For this review, take the finished solid that the model builds, in its own axes (mm). A direction names the side the tool comes from. Coordinates: 2 decimals unless noted, no trailing zeros. Loops run counter-clockwise (first coordinate to the right, second up) from the corner with the lowest first, then second, coordinate; pieces in that order, holes last. Notation, with made-up numbers: M -32.75,52.5 L 3.25,52.5 A3 ccw 3.25,56.5 Z; hole C -12,2.25 d2. An arc over 180 degrees is marked long. Write item = value, one per line.
from build123d import *

# Parameters (mm, degrees)
SKETCH_1_W          = 5.6
SKETCH_1_H          = 10
EXTRUDE_1_DEPTH     = 8
SKETCH_2_W          = 3.1
SKETCH_2_H          = 5.5
CUT_EXTRUDE_1_DEPTH = 11.970870522
CUT_EXTRUDE_2_REACH = 15.109
SKETCH_3_R          = 1.5
SKETCH_4_R          = 1.5
CUT_EXTRUDE_3_DEPTH = 11.970870522
FILLET_1_R          = 3


with BuildPart() as part:
    # 草图1 → 凸台-拉伸1 (new body)
    with BuildSketch(Plane(origin=(0, 0, 0), x_dir=(1, 0, 0), z_dir=(0, 1, 0))):
        Rectangle(SKETCH_1_W, SKETCH_1_H)
    extrude(amount=EXTRUDE_1_DEPTH)

    # 草图2 → 切除-拉伸1 (cut, through all)
    with BuildSketch(Plane(origin=(2.8, 0, 0), x_dir=(0, 0, -1), z_dir=(1, 0, 0))):
        with Locations((-1, 4)):
            Rectangle(SKETCH_2_W, SKETCH_2_H)
    extrude(amount=-CUT_EXTRUDE_1_DEPTH, mode=Mode.SUBTRACT)

    # 草图3 → 切除-拉伸2 (cut, up to next)
    with BuildSketch(Plane.XY.offset(5), mode=Mode.PRIVATE) as cut_extrude_2_sk1:
        with Locations((0, 4)):
            Circle(SKETCH_3_R)
    cut_extrude_2_tool1 = extrude(cut_extrude_2_sk1.sketch, amount=-CUT_EXTRUDE_2_REACH, mode=Mode.PRIVATE) & part.part
    # 草图3 → 切除-拉伸2 (cut, up to next)
    with BuildSketch(Plane.XY.offset(5), mode=Mode.PRIVATE) as cut_extrude_2_sk2:
        with BuildLine():
            Line((2.8, 5.5), (0, 5.5))
            ThreePointArc((0, 5.5), (1.060660172, 5.060660172), (1.5, 4))
            ThreePointArc((1.5, 4), (1.060660172, 2.939339828), (0, 2.5))
            Line((0, 2.5), (2.8, 2.5))
            Line((2.8, 2.5), (2.8, 5.5))
        make_face()
    cut_extrude_2_tool2 = extrude(cut_extrude_2_sk2.sketch, amount=-CUT_EXTRUDE_2_REACH, mode=Mode.PRIVATE) & part.part
    add(cut_extrude_2_tool1.solids().sort_by_distance((0, 4, 5))[0], mode=Mode.SUBTRACT)
    add(cut_extrude_2_tool2.solids().sort_by_distance((1.954494, 4, 5))[0], mode=Mode.SUBTRACT)

    # 草图4 → 切除-拉伸3 (cut, through all)
    with BuildSketch(Plane(origin=(2.8, 0, 0), x_dir=(0, 0, -1), z_dir=(1, 0, 0))):
        with Locations((3, 4)):
            Circle(SKETCH_4_R)
    extrude(amount=-CUT_EXTRUDE_3_DEPTH, mode=Mode.SUBTRACT)

    # 圆角1
    fillet_1_edges = [part.edges().sort_by_distance(p)[0] for p in [
        (0, 8, -5),
        (0, 0, -5),
    ]]
    fillet(fillet_1_edges, radius=FILLET_1_R)


solid = part.part
Q1. Add section C-C (z = 1). Write out the cut boundary in (x, y), and give its area (3 significant figures).
Solved:
outline = M -2.8,0 L 2.8,0 L 2.8,1.25 L -2.8,1.25 Z; M -2.8,6.75 L 2.8,6.75 L 2.8,8 L -2.8,8 Z
area = 14.0 mm²
Q2. Add section D-D (y = 2). Write out the cut boundary in (x, z), and give its area (3 significant figures).
Solved:
outline = M -2.8,-4.83 L 2.8,-4.83 L 2.8,-0.55 L -2.8,-0.55 Z; M -2.8,2.55 L 2.8,2.55 L 2.8,5 L -2.8,5 Z
area = 37.7 mm²
Q3. Draft analysis for pull direction Y (two halves, no side actions). For faces 4 (the face through (0, 6.75, 1)), 5 (the face through (0, 0, 1)), 6 (the face through (-2, 4, 5)), 7 (the face through (1, 2.5, 4)), state which applies: +Y half, -Y half, draft (parallel to the pull), parting line (faces both ways), or undercut.
Solved:
face_4 = undercut
face_5 = -Y half
face_6 = draft
face_7 = undercut
Q4. Add section A-A (x = -2.15). Write out the cut boundary in (y, z), and give its area (3 significant figures).
Solved:
outline = M 0,-2 A3 ccw 3,-5 L 5,-5 A3 ccw 8,-2 L 8,5 L 0,5 Z; hole M 1.25,-0.55 L 6.75,-0.55 L 6.75,2.55 L 1.25,2.55 Z; hole C 4,-3 d3
area = 52.0 mm²
Q5. For line 1 along Y through (x, z) = (1.6, 2.5); line 2 along Z through (x, y) = (-1.95, 4.75); line 3 along Y through (x, z) = (-0.5, -3), list the stretches that pass through material, from the lowest coordinate up.
Solved:
line_1 = 0 to 1.25, 6.75 to 8
line_2 = -5 to -4.3, -1.7 to -0.55, 2.55 to 5
line_3 = 0.17 to 2.5, 5.5 to 7.83
Q6. Add section B-B (y = 4). Write out the cut boundary in (x, z).
Solved:
outline = M -2.8,-5 L 2.8,-5 L 2.8,-4.5 L -2.8,-4.5 Z; M -2.8,-1.5 L 2.8,-1.5 L 2.8,-0.55 L -2.8,-0.55 Z; M -2.8,2.55 L -1.5,2.55 L -1.5,5 L -2.8,5 Z
Q7. Machinability: for faces 1 (the face through (1, 5.5, 4)), 2 (the face through (0, 4, -0.55)), 3 (the face through (0.04, 7.14, -4.1)), which of the approach directions +Z, -Z, +X, -X, +Y, -Y give a long, thin tool a straight path to every point of the face, cutting with its end or side? Answer none if there is none.
Solved:
face_1 = +Z, +X
face_2 = +X, -X
face_3 = -Z, +X, -X, +Y
Q8. For pin 1 Ø1.5 at (x, y) = (-2, 7) entering from -Z, flat-tipped, find the tip position at first contact; note if it passes through.
Solved:
pin_1 = -4.73
